from build123d import *

# Parameters (mm, degrees)
F0_W     = 91.8421666365
F0_H     = 93.1266715601
F0_R     = 26.25
F1_DEPTH = 6
F2_R     = 42.5
F2_R_2   = 26.25
F3_DEPTH = 25
F4_SIZE  = 15


with BuildPart() as f1:
    # F0 (on Top) → F1 (new body)
    with BuildSketch(Plane.XY):
        Rectangle(F0_W, F0_H)
        Circle(F0_R, mode=Mode.SUBTRACT)
    extrude(amount=F1_DEPTH)

    # F2 (on face) → F3 (join)
    with BuildSketch(Plane.XY.offset(6)):
        Circle(F2_R)
        Circle(F2_R_2, mode=Mode.SUBTRACT)
    extrude(amount=F3_DEPTH)

    # F4
    f4_edges = [f1.edges().sort_by_distance(p)[0] for p in [
        (-26.25, 0, 31),
    ]]
    chamfer(f4_edges, length=F4_SIZE)


solid = f1.part
The listing builds one solid part. Answer for the finished solid, in the listing's coordinates (mm). A direction names the side the tool comes from. Coordinates: 2 decimals unless noted, no trailing zeros. Loops run counter-clockwise (first coordinate to the right, second up) from the corner with the lowest first, then second, coordinate; pieces in that order, holes last. Notation, with made-up numbers: (-18, 86) -> (29, 86) arc R19 ccw to (29, 120) -> close; hole circle Ø7 at (-33.5, 3.25). An arc over 180 degrees is marked (long way). Answer in a Markdown table with one row per item. Add a question column.
1. For faces 4 (the flat face through (-1, -46.563, 3)), 5 (the cylindrical face through (-33.727, -25.861, 18.325)), determine the directions among +Z, -Z, +X, -X, +Y, -Y from which every point of the face is accessible in a straight line to the end or side of a thin tool.
2. The part is cut by section A-A, the plane x = 0. Write down the section's boundary in (y, z).
3. Determine the mould class of faces 1 (the conical face through (12.449, -23.934, 16.728)), 2 (the flat face through (45.921, -1, 3)), 3 (the flat face through (-41, 6, 31)) for opening direction X: +X half, -X half, draft (parallel to the pull), parting line (faces both ways), or undercut.
4. Consider line 1 (Y direction, x = 0, z = 4.5); line 2 (Y direction, x = 0, z = 8); line 3 (Z direction, x = 31.5, y = -31.5). Determine where each line is inside the solid, lowest interval first. Write a range as [from, to].
5. Flat-ended cylindrical pins translate along their axes: P1, Ø5, axis at y = 21, z = 27, coming from the -X side; P2, Ø1.5, axis at y = 27, z = 26, coming from the +X side; P3, Ø1.5, axis at x = 23, z = 27.5, coming from the +Y side. Find the tip coordinate at first contact, or state that the pin passes through.
6. The part is cut by section D-D, the plane z = 13.5. Write down the section's boundary in (x, y), then the cut area to 3 significant figures.
7. The part is cut by section B-B, the plane y = 0. Write down the section's boundary in (x, z).
8. The part is cut by section C-C, the plane z = 19. Write down the section's boundary in (x, y).
Answer below:
| question | item | result |
|---|---|---|
| 1 | face 4 | +Z, -Z, +X, -X, -Y |
| 1 | face 5 | +Z |
| 2 | outline | (-46.56, 0) -> (-26.25, 0) -> (-26.25, 16) -> (-41.25, 31) -> (-42.5, 31) -> (-42.5, 6) -> (-46.56, 6) -> close; (26.25, 0) -> (46.56, 0) -> (46.56, 6) -> (42.5, 6) -> (42.5, 31) -> (41.25, 31) -> (26.25, 16) -> close |
| 3 | face 1 | undercut |
| 3 | face 2 | +X half |
| 3 | face 3 | draft |
| 4 | line 1 | [-46.56, -26.25], [26.25, 46.56] |
| 4 | line 2 | [-42.5, -26.25], [26.25, 42.5] |
| 4 | line 3 | [0, 6] |
| 5 | P1 | x = -38.26 |
| 5 | P2 | x = 33.42 |
| 5 | P3 | y = 36.21 |
| 6 | outline | circle Ø85 at (0, 0); hole circle Ø52.5 at (0, 0) |
| 6 | area | 3,510 mm2 |
| 7 | outline | (-45.92, 0) -> (-26.25, 0) -> (-26.25, 16) -> (-41.25, 31) -> (-42.5, 31) -> (-42.5, 6) -> (-45.92, 6) -> close; (26.25, 0) -> (45.92, 0) -> (45.92, 6) -> (42.5, 6) -> (42.5, 31) -> (41.25, 31) -> (26.25, 16) -> close |
| 8 | outline | circle Ø85 at (0, 0); hole circle Ø58.5 at (0, 0) |
